from build123d import *

# Parameters (mm, degrees)
CUT_EXTRUDE1_DEPTH = 7.366
CIRPATTERN1_COUNT  = 36
SKETCH5_R          = 1.27
CUT_EXTRUDE2_DEPTH = 22.86


with BuildPart() as part:
    # Sketch2 → Revolve1 (revolve)
    with BuildSketch(Plane.XY):
        Polygon((-6.223, 2.794), (6.223, 2.794), (6.223, 14.56436), (3.683, 14.56436), (3.683, 11.64336), (-3.683, 11.64336), (-3.683, 14.56436), (-6.223, 14.56436), align=None)
    revolve(axis=Axis((-20.14780731, 0, 0), (1, 0, 0)))

    # Sketch3 → Cut-Extrude1 (cut)
    with BuildSketch(Plane.ZY.offset(-3.683)):
        Polygon((-1.27, 11.64336), (-0.9779, 10.11936), (-0.2921, 10.11936), (0, 11.64336), align=None)
    cut_extrude1 = extrude(amount=CUT_EXTRUDE1_DEPTH, mode=Mode.SUBTRACT)

    # CirPattern1: Cut-Extrude1 ×36 about axis
    cirpattern1_axis = Axis((0, 0, 0), (1, 0, 0))
    for i in range(1, CIRPATTERN1_COUNT):
        add(cut_extrude1.rotate(cirpattern1_axis, i * 360 / CIRPATTERN1_COUNT), mode=Mode.SUBTRACT)

    # Sketch5 → Cut-Extrude2 (cut)
    with BuildSketch(Plane.ZY.offset(6.223)):
        with Locations((0, 4.8895)):
            Circle(SKETCH5_R)
        with Locations((0, -4.8895)):
            Circle(SKETCH5_R)
    extrude(amount=-CUT_EXTRUDE2_DEPTH, mode=Mode.SUBTRACT)


solid = part.part
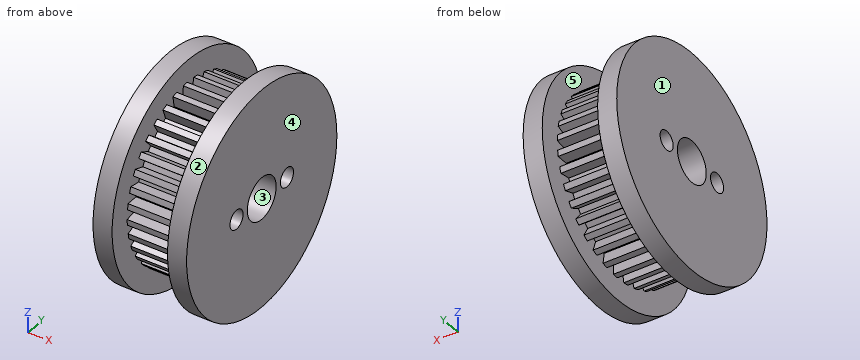
The listing builds one solid part. Answer for the finished solid, in the listing's coordinates (mm). Face numbers are marked on the shaded views. A direction names the side the tool comes from. Give positions to 0.01 mm unless a question says otherwise; leave off trailing zeros.
Item 1: Determine the mould class of the marked faces 1, 2 and 3 for opening direction Y: released by +Y, released by -Y, zero draft, split by the parting line, or undercut.
Item 2: Flat-ended cylindrical pins translate along their axes: P1, Ø4, axis at x = -1.5, y = -1, coming from the +Z side; P2, Ø2, axis at x = -3.5, y = -1.5, coming from the +Z side; P3, Ø6, axis at x = 1.5, z = -4, coming from the +Y side; P4, Ø2, axis at y = -4.89, z = 0, coming from the -X side. Find the tip coordinate at first contact, or state that the pin passes through.
Item 3: Which of the six approach directions +Z, -Z, +X, -X, +Y, -Y give full straight-line access (tool end or side, diameter ignored) to the marked faces 4 and 5?
Item 4: Section A-A, the plane x = 0.25 is taken. Count the separate pieces of the cut face and the enclosed holes in it, plus the area to 3 significant figures.
Item 5: Find the intervals of material crossed by line 1 along X through (y, z) = (-13, -3.5); line 2 along Z through (x, y) = (-0.75, -8.75); line 3 along Z through (x, y) = (-0.25, -10.5), in increasing order.
Completed:
1. face 1: zero draft
1. face 2: split by the parting line
1. face 3: undercut
2. P1: stops at z = 11.64
2. P2: stops at z = 14.56
2. P3: stops at y = 14.43
2. P4: passes through
3. face 4: +Z, -Z, +X, +Y, -Y
3. face 5: none
4. separate pieces: 1
4. enclosed holes: 3
4. area: 339 mm2
5. line 1: x = -6.22 to -3.68, 3.68 to 6.22
5. line 2: z = -7.68 to -7.28, -5.96 to 5.36, 6.32 to 7.39
5. line 3: z = -4.65 to -3.72, -2.65 to -1.65, -0.79 to 0.22, 1.05 to 2.04, 2.99 to 3.91
